Read the model definition and answer for the solid it produces. Units are mm, in the model's axes. Coordinates: 2 decimals unless noted, no trailing zeros. Write each loop counter-clockwise with the first axis right and the second up, starting at its lowest first coordinate (ties: lowest second). Pieces come first, ordered by that corner, then holes. Notation, with made-up numbers: (-12, 34) -> (21, 34) arc R31 ccw to (21, 71) -> close; hole circle Ø6 at (-6.75, 45.5). An arc over 180 degrees is marked (long way). One line per item, written item: value. Start each with the question number.
1. For a pull along Y with two mould halves and no side action, classify faces 1 (the cylindrical face through (24.77, 61.68, 0.79)), 2 (the flat face through (7, 15, 1.6)), 3 (the cylindrical face through (-21.862, 46.183, 0.789)) as pulls with the +Y half, pulls with the -Y half, needs draft (parallel to the pull), parting line crosses it, or undercut.
2. Find section A-A, the plane x = 0. Write down the section's boundary in (y, z), and give its area (3 significant figures).
3. Given P1, Ø0.5, axis at x = -13, z = 0.5, coming from the -Y side; P2, Ø0.8, axis at y = 23, z = 1, coming from the +X side, each flat-ended and moving along its own axis, determine where each tip first touches the part or whether it passes through.
4. Find section B-B, the plane x = -25. Write down the section's boundary in (y, z).
5. Find section D-D, the plane y = 0. Write down the section's boundary in (x, z).
6. Find section C-C, the plane z = 1.35. Write down the section's boundary in (x, y).
7. Consider line 1 along X through (y, z) = (40, 1.2); line 2 along Y through (x, z) = (0, 0.9); line 3 along X through (y, z) = (37, 1). Determine where each line is inside the solid, lowest interval first.
```python
from build123d import *

# Parameters (mm, degrees)
SKETCH_R   = 8
SKETCH_R_2 = 3.2
SKETCH_R_3 = 4
SKETCH_R_4 = 1.8
PAD_DEPTH  = 1.6


with BuildPart() as part:
    # Sketch → Pad (new body)
    with BuildSketch(Plane.XY):
        with BuildLine():
            ThreePointArc((-15.710509, 39.895164), (-22, 46.184654), (-28.289491, 39.895164))
            Line((-28.289491, 39.895164), (-30, 39.895164))
            Line((-30, 39.895164), (-30, 64.895162))
            Line((-30, 64.895162), (30, 64.895162))
            Line((30, 33.895162), (30, 64.895162))
            Line((30, 33.895162), (18, 33.895162))
            Line((18, 33.895162), (18, 15.895162))
            Line((18, 15.895162), (30, 15.895162))
            Line((30, 15.895162), (30, -65.104838))
            Line((30, -65.104838), (-12, -65.104838))
            Line((-12, -49.414836), (-12, -65.104838))
            Line((23, -49.414836), (-12, -49.414836))
            Line((23, -8.104836), (23, -49.414836))
            Line((3.490575, -8.104836), (23, -8.104836))
            Line((-3.490575, -8.104836), (3.490575, -8.104836))
            Line((-12, -8.104836), (-3.490575, -8.104836))
            Line((-12, 39.895164), (-12, -8.104836))
            Line((-15.710509, 39.895164), (-12, 39.895164))
        make_face()
        with Locations((0, 39.895164)):
            Circle(SKETCH_R, mode=Mode.SUBTRACT)
        with Locations((22, 39.895164)):
            Circle(SKETCH_R_2, mode=Mode.SUBTRACT)
        with Locations((0, -60.104838)):
            Circle(SKETCH_R_3, mode=Mode.SUBTRACT)
        with Locations((25, -54.494838)):
            Circle(SKETCH_R_4, mode=Mode.SUBTRACT)
        with Locations((25, 59.895164)):
            Circle(SKETCH_R_4, mode=Mode.SUBTRACT)
        with Locations((-25, 59.895162)):
            Circle(SKETCH_R_4, mode=Mode.SUBTRACT)
    extrude(amount=PAD_DEPTH)


solid = part.part
```
Answer block:
1. face 1: undercut
1. face 2: needs draft
1. face 3: pulls with the -Y half
2. outline: (-65.1, 0) -> (-64.1, 0) -> (-64.1, 1.6) -> (-65.1, 1.6) -> close; (-56.1, 0) -> (-49.41, 0) -> (-49.41, 1.6) -> (-56.1, 1.6) -> close; (-8.1, 0) -> (31.9, 0) -> (31.9, 1.6) -> (-8.1, 1.6) -> close; (47.9, 0) -> (64.9, 0) -> (64.9, 1.6) -> (47.9, 1.6) -> close
2. area: 104 mm2
3. P1: stops at y = 39.9
3. P2: stops at x = 18
4. outline: (45.42, 0) -> (58.1, 0) -> (58.1, 1.6) -> (45.42, 1.6) -> close; (61.7, 0) -> (64.9, 0) -> (64.9, 1.6) -> (61.7, 1.6) -> close
5. outline: (-12, 0) -> (30, 0) -> (30, 1.6) -> (-12, 1.6) -> close
6. outline: (-30, 39.9) -> (-28.29, 39.9) arc R6.29 cw to (-15.71, 39.9) -> (-12, 39.9) -> (-12, -8.1) -> (23, -8.1) -> (23, -49.41) -> (-12, -49.41) -> (-12, -65.1) -> (30, -65.1) -> (30, 15.9) -> (18, 15.9) -> (18, 33.9) -> (30, 33.9) -> (30, 64.9) -> (-30, 64.9) -> close; hole circle Ø3.6 at (-25, 59.9); hole circle Ø16 at (0, 39.9); hole circle Ø8 at (0, -60.1); hole circle Ø6.4 at (22, 39.9); hole circle Ø3.6 at (25, -54.49); hole circle Ø3.6 at (25, 59.9)
7. line 1: x = -30 to -28.29, -15.71 to -8, 8 to 18.8, 25.2 to 30
7. line 2: y = -65.1 to -64.1, -56.1 to -49.41, -8.1 to 31.9, 47.9 to 64.9
7. line 3: x = -12 to -7.46, 7.46 to 20.64, 23.36 to 30
